Check sheet for the modelled part. Datum: model origin and axes. Units: mm. Face numbers are marked on the shaded views. A direction names the side the tool comes from. Coordinates: 2 decimals unless noted, no trailing zeros. Order: outer loops, then holes, each group sorted by start corner. A loop starts at its lowest first (then second) coordinate and runs counter-clockwise, first axis right, second up.
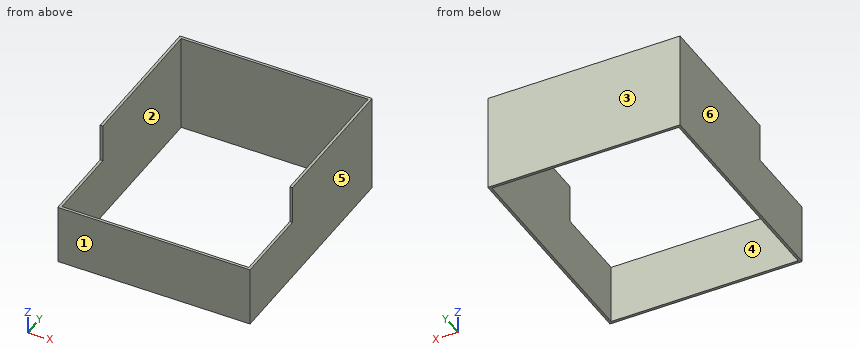
from build123d import *

# Parameters (mm, degrees)
F0_W     = 71.8
F0_H     = 84.6
F2_DEPTH = 36.6
F3_DEPTH = 2
F1_W     = 69.8
F1_H     = 82.6
F4_DEPTH = 36.6
F5_W     = 29.4
F5_H     = 14.3
F6_DEPTH = 71.8


with BuildPart() as f2:
    # F0 (on Top) → F2 (new body)
    with BuildSketch(Plane.XY):
        Rectangle(F0_W, F0_H)
    extrude(amount=F2_DEPTH)

    # F0 (on Top) → F3 (join)
    with BuildSketch(Plane.XY):
        Rectangle(F0_W, F0_H)
    extrude(amount=F3_DEPTH)

    # F1 (on face) → F4 (cut)
    with BuildSketch(Plane.XY):
        Rectangle(F1_W, F1_H)
    extrude(amount=F4_DEPTH, mode=Mode.SUBTRACT)

    # F5 (on face) → F6 (cut)
    with BuildSketch(Plane.YZ.offset(35.9)):
        with Locations((-27.6, 29.45)):
            Rectangle(F5_W, F5_H)
    extrude(amount=-F6_DEPTH, mode=Mode.SUBTRACT)


solid = f2.part
(1) Cross-section at A-A (x = 16). Enter the section's corners in (y, z), and give its area (3 significant figures).
Filled in:
outline: (-42.3, 0) - (-41.3, 0) - (-41.3, 22.3) - (-42.3, 22.3) - close; (41.3, 0) - (42.3, 0) - (42.3, 36.6) - (41.3, 36.6) - close
area: 58.9 mm2
(2) Cross-section at C-C (y = -8). Enter the section's corners in (x, z), and give its area (3 significant figures).
Filled in:
outline: (-35.9, 0) - (-34.9, 0) - (-34.9, 36.6) - (-35.9, 36.6) - close; (34.9, 0) - (35.9, 0) - (35.9, 36.6) - (34.9, 36.6) - close
area: 73.2 mm2
(3) Go/stop test with flat-tipped pins: P1, Ø3, axis at x = 20, z = 26.5, coming from the -Y side; P2, Ø0.8, axis at x = 35.5, z = 32, coming from the -Y side. Record where each tip stops, or that it passes through.
Filled in:
P1: stops at y = 41.3
P2: stops at y = -12.9
(4) Thickness scan on probe 1 along Y at (x, z) = (-24.5, 19); probe 2 along X at (y, z) = (18.5, 11.5); probe 3 along Y at (x, z) = (-6, 30). Record the ranges inside material, lowest first.
Filled in:
probe 1: y = -42.3 to -41.3, 41.3 to 42.3
probe 2: x = -35.9 to -34.9, 34.9 to 35.9
probe 3: y = 41.3 to 42.3
(5) Tool access check on the marked faces 1 and 2. Record the directions out of +Z, -Z, +X, -X, +Y, -Y that give a thin tool (end or side, any length) a straight path to the whole face; none if there is none.
Filled in:
face 1: +Z, -Z, +X, -X, -Y
face 2: +Z, -Z
(6) Cross-section at B-B (z = 21). Enter the section's corners in (x, y), and give its area (3 significant figures).
Filled in:
outline: (-35.9, -42.3) - (35.9, -42.3) - (35.9, 42.3) - (-35.9, 42.3) - close; hole (-34.9, -41.3) - (34.9, -41.3) - (34.9, 41.3) - (-34.9, 41.3) - close
area: 309 mm2
(7) Release check for a two-part mould opening along X. For the marked faces 3, 4, 5 and 6 record: +X half, -X half, draft (parallel to the pull), parting line (faces both ways), or undercut.
Filled in:
face 3: draft
face 4: undercut
face 5: +X half
face 6: -X half
